Could you check a few things on this model? Use its own coordinates, in mm. Face numbers are marked on the shaded views. A direction names the side the tool comes from. Coordinates: 2 decimals unless noted, no trailing zeros. Loops run counter-clockwise (first coordinate to the right, second up) from the corner with the lowest first, then second, coordinate; pieces in that order, holes last. Notation, with made-up numbers: (72.25, 85) - (129.25, 85) arc R32 ccw to (129.25, 120) - close; hole circle Ø11 at (78, 87). An arc over 180 degrees is marked (long way). Use CSV: the item, a comma, the result in double quotes.
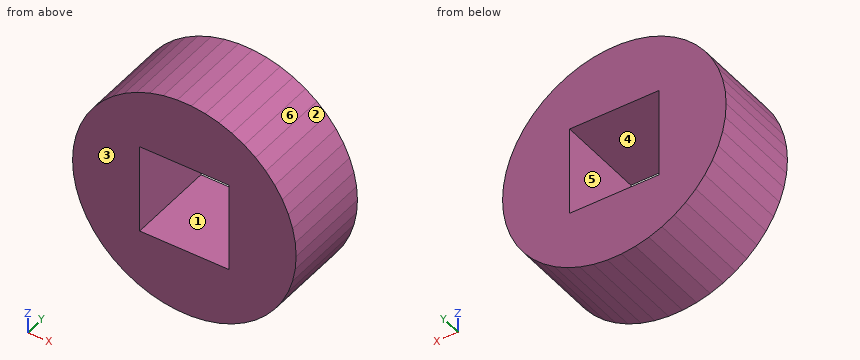
from build123d import *

# Parameters (mm, degrees)
F1_DEPTH = 50.8
F3_DEPTH = 76.2


with BuildPart() as f1:
    # F0 (on Front) → F1 (new body)
    with BuildSketch(Plane.XZ):
        Polygon((3.987198, 63.374697), (-3.987198, 63.374697), (-11.898713, 62.37524), (-19.622579, 60.392089), (-27.036985, 57.456518), (-34.025001, 53.614823), (-40.476423, 48.927591), (-46.289508, 43.468741), (-51.372579, 37.324364), (-55.645474, 30.591358), (-59.040807, 23.375909), (-61.505031, 15.791808), (-62.999284, 7.95866), (-63.5, 0), (-62.999284, -7.95866), (-61.505031, -15.791808), (-59.040807, -23.375909), (-55.645474, -30.591358), (-51.372579, -37.324364), (-46.289508, -43.468741), (-40.476423, -48.927591), (-34.025001, -53.614823), (-27.036985, -57.456518), (-19.622579, -60.392089), (-11.898713, -62.37524), (-3.987198, -63.374697), (3.987198, -63.374697), (11.898713, -62.37524), (19.622579, -60.392089), (27.036985, -57.456518), (34.025001, -53.614823), (40.476423, -48.927591), (46.289508, -43.468741), (51.372579, -37.324364), (55.645474, -30.591358), (59.040807, -23.375909), (61.505031, -15.791808), (62.999284, -7.95866), (63.5, 0), (62.999284, 7.95866), (61.505031, 15.791808), (59.040807, 23.375909), (55.645474, 30.591358), (51.372579, 37.324364), (46.289508, 43.468741), (40.476423, 48.927591), (34.025001, 53.614823), (27.036985, 57.456518), (19.622579, 60.392089), (11.898713, 62.37524), align=None)
    extrude(amount=F1_DEPTH)

    # F2 (on face) → F3 (cut)
    with BuildSketch(Plane.XZ.offset(50.8)):
        Polygon((25.4, 25.4), (0, 25.4), (-25.4, 25.4), (-25.4, 0), (-25.4, -25.4), (0, -25.4), (25.4, -25.4), (25.4, 0), align=None)
    extrude(amount=-F3_DEPTH, mode=Mode.SUBTRACT)


solid = f1.part
(1) Thinking about a two-plate mould opening in X: for the marked faces 1, 2, 3 and 4, which applies, +X half, -X half, draft (parallel to the pull), parting line (faces both ways), or undercut?
Computed:
face 1,"undercut"
face 2,"+X half"
face 3,"draft"
face 4,"undercut"
(2) Suppose I cut it at D-D (z = -32.5). Write out the boundary of the cut face in (x, y), plus the area to 3 significant figures.
Computed:
outline,"(-54.43, -50.8) - (54.43, -50.8) - (54.43, 0) - (-54.43, 0) - close"
area,"5,530 mm²"
(3) Suppose I cut it at C-C (x = -36). Write out the boundary of the cut face in (y, z), plus the area to 3 significant figures.
Computed:
outline,"(-50.8, -52.18) - (0, -52.18) - (0, 52.18) - (-50.8, 52.18) - close"
area,"5,300 mm²"
(4) Which directions (+Z, -Z, +X, -X, +Y, -Y) give clear straight access to the entire face, cutting with the end or side of a thin tool? Please do the marked faces 5 and 6.
Computed:
face 5,"+Y, -Y"
face 6,"+Z, +X, +Y, -Y"
(5) Suppose I cut it at B-B (z = 11). Write out the boundary of the cut face in (x, y).
Computed:
outline,"(-62.42, -50.8) - (-25.4, -50.8) - (-25.4, 0) - (-62.42, 0) - close; (25.4, -50.8) - (62.42, -50.8) - (62.42, 0) - (25.4, 0) - close"
(6) Please list where these lines run through material, in increasing order: line 1 (X direction, y = -28.5, z = -2.5); line 2 (Z direction, x = -1, y = -4); line 3 (X direction, y = -23, z = 24.5).
Computed:
line 1,"x = -63.34 to -25.4, 25.4 to 63.34"
line 2,"z = -63.37 to -25.4, 25.4 to 63.37"
line 3,"x = -58.51 to -25.4, 25.4 to 58.51"
(7) Suppose I cut it at A-A (x = -1). Write out the boundary of the cut face in (y, z).
Computed:
outline,"(-50.8, -63.37) - (0, -63.37) - (0, -25.4) - (-50.8, -25.4) - close; (-50.8, 25.4) - (0, 25.4) - (0, 63.37) - (-50.8, 63.37) - close"
(8) Will these pins go through, and if not, where does the flat tip stop? pin 1 (4 mm diameter, centred on y = -25.5, z = -35, fed in from +X); pin 2 (2 mm diameter, centred on y = -23.5, z = 25.5, fed in from -X); pin 3 (8 mm diameter, centred on x = -20.5, z = -19, fed in from +Y); pin 4 (10 mm diameter, centred on x = -49.5, y = -45, fed in from +Z).
Computed:
pin 1,"stops at x = 54.12"
pin 2,"stops at x = -58.51"
pin 3,"passes through"
pin 4,"stops at z = 45.15"
